Geometry: final body of the model. Coordinates: model frame, mm. A direction names the side the tool comes from. Coordinates: 2 decimals unless noted, no trailing zeros. Write each loop counter-clockwise with the first axis right and the second up, starting at its lowest first coordinate (ties: lowest second). Pieces come first, ordered by that corner, then holes. Notation, with made-up numbers: (-34.5, 64) -> (0.5, 64) arc R11 cw to (0.5, 81) -> close; hole circle Ø10 at (-27.5, -36.5). An arc over 180 degrees is marked (long way). Answer as a JSON object with one key per item and string values. Group by question number.
```python
from build123d import *

# Parameters (mm, degrees)
SALIENTE_EXTRUIR1_DEPTH = 76.2
CROQUIS2_W              = 5
CROQUIS2_H              = 76.2
CORTAR_EXTRUIR1_DEPTH   = 76.2


with BuildPart() as part:
    # Croquis1 → Saliente-Extruir1 (new body)
    with BuildSketch(Plane.XY):
        Polygon((0, 0), (650, 0), (478.989928337, 469.846310393), (171.010071663, 469.846310393), align=None)
        Polygon((188.795343133, 444.446310393), (461.204656867, 444.446310393), (613.725040629, 25.4), (36.274959371, 25.4), align=None, mode=Mode.SUBTRACT)
    extrude(amount=SALIENTE_EXTRUIR1_DEPTH)

    # Croquis2 → Cortar-Extruir1 (cut)
    with BuildSketch(Plane.XZ):
        with Locations((2.5, 38.1)):
            Rectangle(CROQUIS2_W, CROQUIS2_H)
        with Locations((647.5, 38.1)):
            Rectangle(CROQUIS2_W, CROQUIS2_H)
    extrude(amount=-CORTAR_EXTRUIR1_DEPTH, mode=Mode.SUBTRACT)


solid = part.part
```
Item 1: Ray query, L1, parallel to Y at x = 460, z = 10.5; L2, parallel to X at y = 144, z = 60.5; L3, parallel to X at y = 79.5, z = 31. Return the intervals inside material, ascending. Write a range as [from, to].
Item 2: Mould query, pull axis Y, two halves, no side actions, for faces 3 (the flat face through (5, 7, 38)), 4 (the flat face through (563.157, 238.599, 37.567)), 5 (the flat face through (323, 444.446, 38)). Classes: +Y half, -Y half, draft (parallel to the pull), parting line (faces both ways), or undercut.
Item 3: Section C-C on y = 411. Output: boundary loops of the cut face in (x, z).
Item 4: Section B-B on z = 63. Output: boundary loops of the cut face in (x, y).
Item 5: Contact query for flat-ended pins moving along their axis: pin 1 (10 mm diameter, centred on y = 125, z = 46, fed in from -X); pin 2 (4 mm diameter, centred on y = 67.5, z = 30, fed in from +X); pin 3 (8 mm diameter, centred on y = 67.5, z = 31.5, fed in from -X). Output: stop coordinate, or through.
Item 6: Section A-A on x = 332. Output: boundary loops of the cut face in (y, z), then the cut area to 3 significant figures.
Item 7: Set-up query: faces 1 (the flat face through (89.167, 244.985, 37.567)), 2 (the flat face through (329, 25.4, 38)). Return all of +Z, -Z, +X, -X, +Y, -Y with unobstructed straight access to the full face (end or side cutting, diameter ignored); none if empty.
Answer sheet:
{
 "1": {"L1": "y = [0, 25.4], [444.45, 469.85]", "L2": "x = [52.41, 79.44], [570.56, 597.59]", "L3": "x = [28.94, 55.97], [594.03, 621.06]"},
 "2": {"face 3": "draft", "face 4": "+Y half", "face 5": "undercut"},
 "3": {"outline": "(149.59, 0) -> (176.62, 0) -> (176.62, 76.2) -> (149.59, 76.2) -> close; (473.38, 0) -> (500.41, 0) -> (500.41, 76.2) -> (473.38, 76.2) -> close"},
 "4": {"outline": "(5, 0) -> (645, 0) -> (645, 13.74) -> (478.99, 469.85) -> (171.01, 469.85) -> (5, 13.74) -> close; hole (36.27, 25.4) -> (613.73, 25.4) -> (461.2, 444.45) -> (188.8, 444.45) -> close"},
 "5": {"pin 1": "stops at x = 43.68", "pin 2": "stops at x = 626.16", "pin 3": "stops at x = 23.11"},
 "6": {"outline": "(0, 0) -> (25.4, 0) -> (25.4, 76.2) -> (0, 76.2) -> close; (444.45, 0) -> (469.85, 0) -> (469.85, 76.2) -> (444.45, 76.2) -> close", "area": "3,870 mm^2"},
 "7": {"face 1": "+Z, -Z, -X, +Y", "face 2": "+Z, -Z"}
}
